Here's how the part is built. I have some questions about the finished solid (model axes, mm). Round coordinates to 2 decimals unless told otherwise and drop trailing zeros. Loops run counter-clockwise (first coordinate to the right, second up) from the corner with the lowest first, then second, coordinate; pieces in that order, holes last. Notation, with made-up numbers: M 27.25,-25 L 55.25,-25 A20 cw 55.25,1 Z; hole C 13.5,-38 d4. An arc over 180 degrees is marked long. Answer as a JSON object with one key per item and string values.
Autodesk Inventor part; units mm, degrees
ref_plane "YZ Plane" through (0, 0, 0) normal (1, 0, 0) x (0, 1, 0)
ref_plane "XZ Plane" through (0, 0, 0) normal (0, 1, 0) x (-1, 0, 0)
ref_plane "XY Plane" through (0, 0, 0) normal (0, 0, 1) x (1, 0, 0)
sketch "Sketch1" plane through (0, 0, 0) normal (0, 1, 0) x (-1, 0, 0)
  line L0 (-24, 27.5) -> (24, 27.5)
  line L1 (24, 27.5) -> (24, -27.5)
  line L2 (24, -27.5) -> (-24, -27.5)
  line L3 (-24, -27.5) -> (-24, 27.5)
  dimension "d13" = 48
  dimension "d14" = 55
extrude "Extrusion1" add sketch "Sketch1" along normal blind 1.5
sketch "Sketch2" plane through (0, 1.5, 0) normal (0, 1, 0) x (1, 0, 0)
  circle A0 centre (19, 21) radius 2.5
  circle A1 centre (19, -21) radius 2.5
  circle A2 centre (-19, -21) radius 2.5
  circle A3 centre (-19, 21) radius 2.5
  circle A4 centre (-13, -15) radius 2.5
  circle A5 centre (13, -15) radius 2.5
  circle A6 centre (13, 15) radius 2.5
  circle A7 centre (-13, 15) radius 2.5
  circle A8 centre (19, -21) radius 1.5
  circle A9 centre (19, 21) radius 1.5
  circle A10 centre (-19, 21) radius 1.5
  circle A11 centre (-19, -21) radius 1.5
  dimension "d47" = 3
  dimension "d48" = 3
  dimension "d50" = 3
extrude "Extrusion2" add sketch "Sketch2" along normal blind 4 contours A0 | A1 | A2 | A3
sketch "Sketch3" plane through (0, 1.5, 0) normal (0, 1, 0) x (1, 0, 0)
  circle A0 centre (-13, -15) radius 2.5
  circle A1 centre (13, -15) radius 2.5
  circle A2 centre (13, 15) radius 2.5
  circle A3 centre (-13, 15) radius 2.5
  point P0 (0, 0)
extrude "Extrusion3" cut sketch "Sketch3" against normal through all
properties part number "Box2_Buttom"
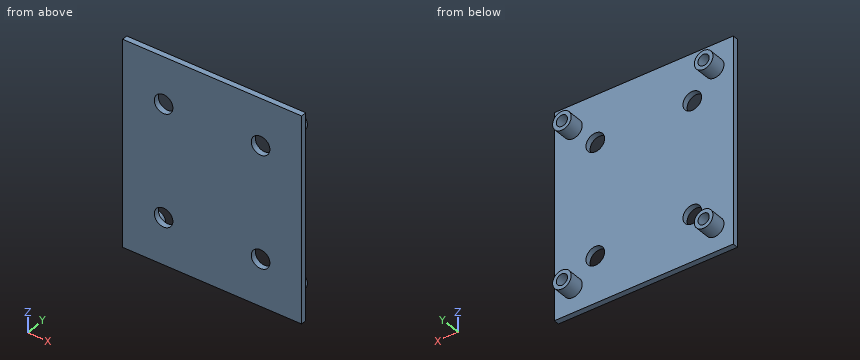
Item 1: I want a section at D-D, the plane x = 19. Please give me the cut outline in (y, z).
Resolved:
{"outline": "M 0,-27.5 L 1.5,-27.5 L 1.5,-23.5 L 5.5,-23.5 L 5.5,-22.5 L 1.5,-22.5 L 1.5,-19.5 L 5.5,-19.5 L 5.5,-18.5 L 1.5,-18.5 L 1.5,18.5 L 5.5,18.5 L 5.5,19.5 L 1.5,19.5 L 1.5,22.5 L 5.5,22.5 L 5.5,23.5 L 1.5,23.5 L 1.5,27.5 L 0,27.5 Z"}
Item 2: I'm going to push flat-ended pins straight in: pin 1 Ø3.5 at (x, z) = (19, -21) entering from +Y; pin 2 Ø24 at (x, z) = (-3, 8.5) entering from +Y; pin 3 Ø1 at (x, y) = (-4.5, 2.5) entering from -Z. Where does each tip first touch, or does it pass through?
Resolved:
{"pin 1": "y = 5.5", "pin 2": "y = 1.5", "pin 3": "through"}
Item 3: Please list where these lines run through material, in increasing order: probe 1 along Z at (x, y) = (-19, 3.6); probe 2 along X at (y, z) = (0.65, 15); probe 3 along X at (y, z) = (2.4, -21). Write a range as from..to.
Resolved:
{"probe 1": "-23.5..-22.5, -19.5..-18.5, 18.5..19.5, 22.5..23.5", "probe 2": "-24..-15.5, -10.5..10.5, 15.5..24", "probe 3": "-21.5..-20.5, -17.5..-16.5, 16.5..17.5, 20.5..21.5"}
Item 4: I want a section at A-A, the plane y = 4.1. Please give me the cut outline in (x, z).
Resolved:
{"outline": "C -19,-21 d5; C -19,21 d5; C 19,-21 d5; C 19,21 d5; hole C -19,-21 d3; hole C -19,21 d3; hole C 19,-21 d3; hole C 19,21 d3"}
Item 5: I want a section at C-C, the plane x = -13. Please give me the cut outline in (y, z), then the cut area to 3 significant figures.
Resolved:
{"outline": "M 0,-27.5 L 1.5,-27.5 L 1.5,-17.5 L 0,-17.5 Z; M 0,-12.5 L 1.5,-12.5 L 1.5,12.5 L 0,12.5 Z; M 0,17.5 L 1.5,17.5 L 1.5,27.5 L 0,27.5 Z", "area": "67.5 mm²"}
Item 6: I want a section at B-B, the plane z = -13.5. Please give me the cut outline in (x, y), then the cut area to 3 significant figures.
Resolved:
{"outline": "M -24,0 L -15,0 L -15,1.5 L -24,1.5 Z; M -11,0 L 11,0 L 11,1.5 L -11,1.5 Z; M 15,0 L 24,0 L 24,1.5 L 15,1.5 Z", "area": "60.0 mm²"}
